Autodesk Inventor part; units mm, degrees
ref_plane "YZ Plane" through (0, 0, 0) normal (1, 0, 0) x (0, 1, 0)
ref_plane "XZ Plane" through (0, 0, 0) normal (0, 1, 0) x (-1, 0, 0)
ref_plane "XY Plane" through (0, 0, 0) normal (0, 0, 1) x (1, 0, 0)
sketch "Sketch1" plane through (0, 0, 0) normal (1, 0, 0) x (0, 1, 0)
  line L0 (127, 254) -> (0, 254)
  line L1 (0, 254) -> (0, 0)
  line L2 (0, 0) -> (127, 0)
  line L3 (127, 0) -> (127, 254)
  circle A0 centre (100.0125, 127) radius 14.2875
  circle A1 centre (100.0125, 127) radius 26.9875
  line L4 (76.2, 254) -> (124.914, 137.4039)
  line L5 (124.914, 116.5961) -> (76.2, 0)
  dimension "d0" = 254
  dimension "d1" = 127
  dimension "d2" = 28.575
  dimension "d3" = 12.7
  dimension "d4" = 127
  dimension "d5" = 76.2
  dimension "d6" = 76.2
extrude "Extrusion1" add sketch "Sketch1" along normal blind 12.7 contours L4 A1 L5 L2 L1 L0 | A1
sketch "Sketch2" plane through (12.7, 0, 0) normal (1, 0, 0) x (0, 0, -1)
  circle A0 centre (-241.3, 12.7) radius 1.7272
  line L0 (-254, 76.2) -> (-254, 0)
  line L1 (-254, 0) -> (0, 0)
  dimension "d9" = 12.7
  dimension "d10" = 12.7
  dimension "d11" = 3.4544
extrude "Extrusion2" cut sketch "Sketch2" against normal through all
pattern_linear "Rectangular Pattern1" count 10 spacing 25.4 along (0, 0, -1) of "Extrusion2"
properties part number "Jeep Plate 2.0" material "Polycarbonate, Smoke"
Geometry check sheet. Reference: the model listing, model coordinates, mm. Round coordinates to 2 decimals unless told otherwise and drop trailing zeros. Write each loop counter-clockwise with the first axis right and the second up, starting at its lowest first coordinate (ties: lowest second). Pieces come first, ordered by that corner, then holes. Notation, with made-up numbers: (-35, -3) - (4, -3) arc R24 cw to (4, 17) - close; hole circle Ø8 at (-30.5, -16.5). An arc over 180 degrees is marked (long way). One line per item, written item: value.
1. Cross-section at B-B on z = 127. Record the boundary of the cut face in (x, y) (3 decimals).
The answers:
outline: (0, 0) - (12.7, 0) - (12.7, 85.725) - (0, 85.725) - close; (0, 114.3) - (12.7, 114.3) - (12.7, 127) - (0, 127) - close
2. Scan lines: L1, parallel to Y at x = 3, z = 114.3; L2, parallel to Y at x = 9.5, z = 165.1; L3, parallel to Y at x = 7.5, z = 190.5. Record each from-to range of solid material in increasing order.
The answers:
L1: y = 0 to 10.97, 14.43 to 93.47, 106.56 to 123.95
L2: y = 0 to 10.97, 14.43 to 113.34
L3: y = 0 to 10.97, 14.43 to 102.73
3. Mould release check, pull along Y, two halves, no side actions. Record for faces 1 (the face through (12.7, 48, 129)), 2 (the face through (6.261, 100.216, 196.518)), 3 (the face through (6.26, 113.64, 122.71)): released by +Y, released by -Y, zero draft, split by the parting line, or undercut.
The answers:
face 1: zero draft
face 2: released by +Y
face 3: undercut
4. Cross-section at C-C on y = 111. Record the boundary of the cut face in (x, z).
The answers:
outline: (0, 83.29) - (12.7, 83.29) - (12.7, 117.87) - (0, 117.87) - close; (0, 136.13) - (12.7, 136.13) - (12.7, 170.71) - (0, 170.71) - close
5. Depth check by flat-ended pin: pin 1 Ø1 at (x, z) = (4, 212.5) entering from +Y; pin 2 Ø3 at (y, z) = (12.7, 12.7) entering from -X; pin 3 Ø3 at (x, z) = (10, 46) entering from +Y. Enter the tip coordinate at first touch or a pass-through.
The answers:
pin 1: stops at y = 93.75
pin 2: passes through
pin 3: stops at y = 96.05
6. Cross-section at D-D on z = 200.5. Record the boundary of the cut face in (x, y), and give its area (3 significant figures).
The answers:
outline: (0, 0) - (12.7, 0) - (12.7, 98.55) - (0, 98.55) - close
area: 1,250 mm^2
7. Cross-section at A-A on x = 9.25. Give the number of separate pieces and of enclosed holes in the cut face, and give its area (3 significant figures).
The answers:
separate pieces: 1
enclosed holes: 11
area: 25,300 mm^2
